from build123d import *

# Parameters (mm, degrees)
F0_W     = 57
F0_H     = 110
F1_DEPTH = 5
F2_D     = 3.3
F3_D     = 4.4


with BuildPart() as f1:
    # F0 (on Top) → F1 (new body)
    with BuildSketch(Plane.XY):
        with Locations((15, 0)):
            Rectangle(F0_W, F0_H)
    extrude(amount=F1_DEPTH)

    # F2 (through all)
    with Locations(Plane(origin=(0, 0, 0), x_dir=(1, 0, 0), z_dir=(0, 0, -1))):
        with Locations((-10, -45), (-10, -30), (10, -30), (10, -45), (-10, 30), (-10, 45), (10, 45), (10, 30)):
            Hole(F2_D / 2)

    # F3 (through all)
    with Locations(Plane(origin=(0, 0, 0), x_dir=(1, 0, 0), z_dir=(0, 0, -1))):
        with Locations((23.5, -40), (38.5, -40), (23.5, 40), (38.5, 40)):
            Hole(F3_D / 2)


solid = f1.part
CAD build for the part. Positions are in the model's coordinates, mm. Coordinates: 2 decimals unless noted, no trailing zeros. Loops run counter-clockwise (first coordinate to the right, second up) from the corner with the lowest first, then second, coordinate; pieces in that order, holes last. Notation, with made-up numbers: (-31.75, 71) - (-22.75, 71) arc R11 ccw to (-22.75, 92) - close; hole circle Ø7 at (17, -22.5). An arc over 180 degrees is marked (long way). Use one line per item in the form item = value. Start each with the question number.
1) Band-saw the part on B-B (x = 10). Give the cut face in (y, z), and give its area (3 significant figures).
2) Band-saw the part on A-A (y = -40). Give the cut face in (x, z).
3) Band-saw the part on D-D (z = 4.1). State how many separate pieces and enclosed holes the cut face has, and give its area (3 significant figures).
4) Two-plate mould, pull along X, no slides. Class faces 1 (the face through (15, 1, 0)), 2 (the face through (-13.5, -1, 2)), 3 (the face through (-9.785, -31.636, 2.535)): +X half, -X half, draft (parallel to the pull), parting line (faces both ways), or undercut.
5) Drill centre lines: L1, parallel to X at y = -45, z = 3.45; L2, parallel to Y at x = -10, z = 1.9; L3, parallel to X at y = 40, z = 3.05. Where is each one in solid material? Low to high. Write a range as from..to.
6) Band-saw the part on C-C (x = 38.5). Give the cut face in (y, z).
Check values:
q1.outline = (-55, 0) - (-46.65, 0) - (-46.65, 5) - (-55, 5) - close; (-43.35, 0) - (-31.65, 0) - (-31.65, 5) - (-43.35, 5) - close; (-28.35, 0) - (28.35, 0) - (28.35, 5) - (-28.35, 5) - close; (31.65, 0) - (43.35, 0) - (43.35, 5) - (31.65, 5) - close; (46.65, 0) - (55, 0) - (55, 5) - (46.65, 5) - close
q1.area = 484 mm2
q2.outline = (-13.5, 0) - (21.3, 0) - (21.3, 5) - (-13.5, 5) - close; (25.7, 0) - (36.3, 0) - (36.3, 5) - (25.7, 5) - close; (40.7, 0) - (43.5, 0) - (43.5, 5) - (40.7, 5) - close
q3.separate_pieces = 1
q3.enclosed_holes = 12
q3.area = 6,140 mm2
q4.face_1 = draft
q4.face_2 = -X half
q4.face_3 = undercut
q5.L1 = -13.5..-11.65, -8.35..8.35, 11.65..43.5
q5.L2 = -55..-46.65, -43.35..-31.65, -28.35..28.35, 31.65..43.35, 46.65..55
q5.L3 = -13.5..21.3, 25.7..36.3, 40.7..43.5
q6.outline = (-55, 0) - (-42.2, 0) - (-42.2, 5) - (-55, 5) - close; (-37.8, 0) - (37.8, 0) - (37.8, 5) - (-37.8, 5) - close; (42.2, 0) - (55, 0) - (55, 5) - (42.2, 5) - close
